from build123d import *

# Parameters (mm, degrees)
CYLINDER_R     = 102
CYLINDER_DEPTH = 80
PAD_DEPTH      = 5
SKETCH008_R    = 1.1
POCKET_DEPTH   = 8


with BuildPart() as cylinder:
    # Cylinder → Cylinder (new body)
    with BuildSketch(Plane(origin=(24, 50, -98), x_dir=(1, 0, 0), z_dir=(0, -1, 0))):
        Circle(CYLINDER_R)
    extrude(amount=CYLINDER_DEPTH)


with BuildPart() as cut:
    # Sketch → Pad (new body)
    with BuildSketch(Plane.XY):
        with BuildLine():
            Line((0.614893, -1.006641), (52.614893, -1.006641))
            ThreePointArc((52.614893, -1.006641), (55.44332, 0.164932), (56.614893, 2.993359))
            Line((56.614893, 2.993359), (56.614893, 34.993359))
            ThreePointArc((56.614893, 34.993359), (55.44332, 37.821786), (52.614893, 38.993359))
            Line((52.614893, 38.993359), (0.614893, 38.993359))
            ThreePointArc((0.614893, 38.993359), (-2.213534, 37.821786), (-3.385107, 34.993359))
            Line((-3.385107, 34.993359), (-3.385107, 2.993359))
            ThreePointArc((-3.385107, 2.993359), (-2.213534, 0.164932), (0.614893, -1.006641))
        make_face()
    extrude(amount=PAD_DEPTH)

    # Sketch008 → Pocket (cut)
    with BuildSketch(Plane(origin=(0, 0, 0), x_dir=(1, 0, 0), z_dir=(0, 0, -1))):
        with Locations((1.8, -4)):
            Circle(SKETCH008_R)
        with Locations((1.8, -13)):
            Circle(SKETCH008_R)
        with Locations((1.8, -24)):
            Circle(SKETCH008_R)
        with Locations((1.8, -33)):
            Circle(SKETCH008_R)
        with Locations((46.2, -4)):
            Circle(SKETCH008_R)
        with Locations((46.2, -13)):
            Circle(SKETCH008_R)
        with Locations((46.2, -24)):
            Circle(SKETCH008_R)
        with Locations((46.2, -33)):
            Circle(SKETCH008_R)
    extrude(amount=-POCKET_DEPTH, mode=Mode.SUBTRACT)

    # Cut: cut Cylinder
    add(cylinder.part, mode=Mode.SUBTRACT)


solid = cut.part
Read the model definition and answer for the solid it produces. Units are mm, in the model's axes. Round coordinates to 2 decimals unless told otherwise and drop trailing zeros. Write each loop counter-clockwise with the first axis right and the second up, starting at its lowest first coordinate (ties: lowest second). Pieces come first, ordered by that corner, then holes.
1. The part is cut by section A-A, the plane z = 2.8. State how many separate pieces and enclosed holes the cut face has, then the cut area to 3 significant figures.
2. Given pin 1 Ø2.5 at (x, y) = (46.2, 4) entering from -Z; pin 2 Ø3 at (x, y) = (46.2, 24) entering from -Z; pin 3 Ø6 at (x, y) = (14, 19) entering from -Z, each flat-ended and moving along its own axis, determine where each tip first touches the part or whether it passes through.
3. The part is cut by section B-B, the plane y = 24. Determine the outline of the cut face in (x, z), then the cut area to 3 significant figures.
4. Straight lines are drawn through the part: L1, parallel to Y at x = 46.2, z = 2.6; L2, parallel to Z at x = 48, y = 17; L3, parallel to Z at x = 36, y = 26. For each, find the intervals that lie inside material, in ascending order.
5. Determine the mould class of faces 1 (the face through (55.41, 0.13, 2.46)), 2 (the face through (47.216, 13.421, 3.126)), 3 (the face through (55.474, 37.791, 2.465)), 4 (the face through (56.615, 19, 2)) for opening direction Y: pulls with the +Y half, pulls with the -Y half, needs draft (parallel to the pull), parting line crosses it, or undercut.
6. The part is cut by section D-D, the plane y = 18. Determine the outline of the cut face in (x, z), then the cut area to 3 significant figures.
7. The part is cut by section C-C, the plane x = 1.8. Determine the outline of the cut face in (y, z), then the cut area to 3 significant figures.
Values:
1. separate pieces: 2
1. enclosed holes: 8
1. area: 1,110 mm2
2. pin 1: stops at z = 1.27
2. pin 2: stops at z = 1.21
2. pin 3: stops at z = 3.17
3. outline: (-3.39, 0.26) arc R102 cw to (0.7, 1.3) - (0.7, 5) - (-3.39, 5) - close; (2.9, 1.79) arc R102 cw to (45.1, 1.79) - (45.1, 5) - (2.9, 5) - close; (47.3, 1.3) arc R102 cw to (52.28, 0) - (56.61, 0) - (56.61, 5) - (47.3, 5) - close
3. area: 133 mm2
4. L1: y = -1.01 to 2.9, 5.1 to 11.9, 14.1 to 22.9, 25.1 to 31.9, 34.1 to 38.99
4. L2: z = 1.14 to 5
4. L3: z = 3.29 to 5
5. face 1: pulls with the -Y half
5. face 2: undercut
5. face 3: pulls with the +Y half
5. face 4: needs draft
6. outline: (-3.39, 0.26) arc R102 cw to (52.28, 0) - (56.61, 0) - (56.61, 5) - (-3.39, 5) - close
6. area: 149 mm2
7. outline: (-1.01, 1.55) - (2.9, 1.55) - (2.9, 5) - (-1.01, 5) - close; (5.1, 1.55) - (11.9, 1.55) - (11.9, 5) - (5.1, 5) - close; (14.1, 1.55) - (22.9, 1.55) - (22.9, 5) - (14.1, 5) - close; (25.1, 1.55) - (31.9, 1.55) - (31.9, 5) - (25.1, 5) - close; (34.1, 1.55) - (38.99, 1.55) - (38.99, 5) - (34.1, 5) - close
7. area: 107 mm2
